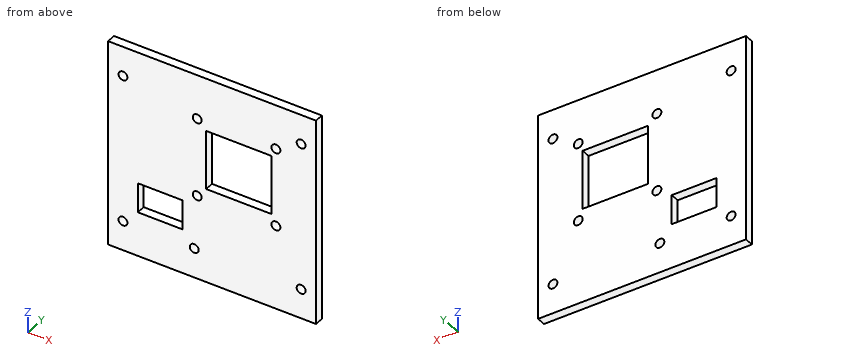
from build123d import *

# Parameters (mm, degrees)
SKETCH1_W           = 70
SKETCH1_H           = 70
BOSS_EXTRUDE1_DEPTH = 3
SKETCH2_R           = 1.5
CUT_EXTRUDE1_DEPTH  = 3
SKETCH3_R           = 1.5
SKETCH3_W           = 15
SKETCH3_H           = 10
SKETCH3_W_2         = 22
SKETCH3_H_2         = 20
CUT_EXTRUDE2_DEPTH  = 3


with BuildPart() as part:
    # Sketch1 → Boss-Extrude1 (new body)
    with BuildSketch(Plane(origin=(0, 0, 0), x_dir=(1, 0, 0), z_dir=(0, 1, 0))):
        Rectangle(SKETCH1_W, SKETCH1_H)
    extrude(amount=BOSS_EXTRUDE1_DEPTH)

    # Sketch2 → Cut-Extrude1 (cut)
    with BuildSketch(Plane(origin=(0, 3, 0), x_dir=(1, 0, 0), z_dir=(0, 1, 0))):
        with Locations(Location((-30, 25, 0), (0, 0, 270))):
            Circle(SKETCH2_R)
        with Locations(Location((30, 25, 0), (0, 0, 90))):
            Circle(SKETCH2_R)
        with Locations(Location((30, -25, 0), (0, 0, 270))):
            Circle(SKETCH2_R)
        with Locations(Location((-30, -25, 0), (0, 0, 90))):
            Circle(SKETCH2_R)
    extrude(amount=-CUT_EXTRUDE1_DEPTH, mode=Mode.SUBTRACT)

    # Sketch3 → Cut-Extrude2 (cut)
    with BuildSketch(Plane(origin=(0, 3, 0), x_dir=(1, 0, 0), z_dir=(0, 1, 0))):
        with Locations(Location((21.5, 6.5, 0), (0, 0, 270))):
            Circle(SKETCH3_R)
        with Locations(Location((21.5, -20, 0), (0, 0, 90))):
            Circle(SKETCH3_R)
        with Locations(Location((-5, -20, 0), (0, 0, 270))):
            Circle(SKETCH3_R)
        with Locations(Location((-6, 25, 0), (0, 0, 270))):
            Circle(SKETCH3_R)
        with Locations(Location((-5, 6.5, 0), (0, 0, 90))):
            Circle(SKETCH3_R)
        with Locations((-17.5, 15)):
            Rectangle(SKETCH3_W, SKETCH3_H)
        with Locations((9, -7)):
            Rectangle(SKETCH3_W_2, SKETCH3_H_2)
    extrude(amount=-CUT_EXTRUDE2_DEPTH, mode=Mode.SUBTRACT)


solid = part.part
CAD build for the part. Positions are in the model's coordinates, mm. Coordinates: 2 decimals unless noted, no trailing zeros. Write each loop counter-clockwise with the first axis right and the second up, starting at its lowest first coordinate (ties: lowest second). Pieces come first, ordered by that corner, then holes. Notation, with made-up numbers: M 58,-34.5 L 95,-34.5 A20 cw 95,-25.5 Z; hole C 54.25,46 d3. An arc over 180 degrees is marked long. Return JSON: item names as keys, results as strings.
Item 1: Slice it at D-D, the plane y = 2.35. State how many separate pieces and enclosed holes the cut face has, and give its area (3 significant figures).
Findings below:
{"separate pieces": "1", "enclosed holes": "11", "area": "4,250 mm2"}
Item 2: Drop a flat-ended pin along its axis: pin 1 Ø1.8 at (x, z) = (-6, -25) entering from +Y. Give the stop position or say it passes through.
Findings below:
{"pin 1": "passes through"}
Item 3: Slice it at C-C, the plane z = -6.5. Write the cut outline in (x, y).
Findings below:
{"outline": "M -35,0 L -6.5,0 L -6.5,3 L -35,3 Z; M -3.5,0 L 20,0 L 20,3 L -3.5,3 Z; M 23,0 L 35,0 L 35,3 L 23,3 Z"}
Item 4: Slice it at B-B, the plane x = -23.5. Write the cut outline in (y, z), and give its area (3 significant figures).
Findings below:
{"outline": "M 0,-35 L 3,-35 L 3,-20 L 0,-20 Z; M 0,-10 L 3,-10 L 3,35 L 0,35 Z", "area": "180 mm2"}
Item 5: Slice it at A-A, the plane z = -17.5. Write the cut outline in (x, y), and give its area (3 significant figures).
Findings below:
{"outline": "M -35,0 L -25,0 L -25,3 L -35,3 Z; M -10,0 L 35,0 L 35,3 L -10,3 Z", "area": "165 mm2"}
Item 6: Probe line 1 (X direction, y = 1.4, z = -6.5); line 2 (X direction, y = 1.9, z = 25); line 3 (X direction, y = 1.9, z = -25). List the from-to ranges inside material, lowest first. Write a range as from..to.
Findings below:
{"line 1": "x = -35..-6.5, -3.5..20, 23..35", "line 2": "x = -35..-31.5, -28.5..28.5, 31.5..35", "line 3": "x = -35..-31.5, -28.5..-7.5, -4.5..28.5, 31.5..35"}
